```python
from build123d import *

# Parameters (mm, degrees)
SKETCH1_R           = 10
BOSS_EXTRUDE1_DEPTH = 2
SKETCH2_R           = 2.5
CUT_EXTRUDE1_DEPTH  = 2
SKETCH3_R           = 1
CUT_EXTRUDE2_DEPTH  = 2


with BuildPart() as part:
    # Sketch1 → Boss-Extrude1 (new body)
    with BuildSketch(Plane(origin=(0, 0, 0), x_dir=(1, 0, 0), z_dir=(0, 1, 0))):
        with Locations(Location((0, 0, 0), (0, 0, 270))):
            Circle(SKETCH1_R)
    extrude(amount=BOSS_EXTRUDE1_DEPTH)

    # Sketch2 → Cut-Extrude1 (cut)
    with BuildSketch(Plane(origin=(0, 2, 0), x_dir=(1, 0, 0), z_dir=(0, 1, 0))):
        with Locations(Location((0, 0, 0), (0, 0, 270))):
            Circle(SKETCH2_R)
    extrude(amount=-CUT_EXTRUDE1_DEPTH, mode=Mode.SUBTRACT)

    # Sketch3 → Cut-Extrude2 (cut)
    with BuildSketch(Plane(origin=(0, 2, 0), x_dir=(1, 0, 0), z_dir=(0, 1, 0))):
        with Locations(Location((7, 0, 0), (0, 0, 270))):
            Circle(SKETCH3_R)
        with Locations(Location((0, -7, 0), (0, 0, 270))):
            Circle(SKETCH3_R)
        with Locations(Location((-7, 0, 0), (0, 0, 270))):
            Circle(SKETCH3_R)
        with Locations(Location((0, 7, 0), (0, 0, 270))):
            Circle(SKETCH3_R)
    extrude(amount=-CUT_EXTRUDE2_DEPTH, mode=Mode.SUBTRACT)


solid = part.part
```
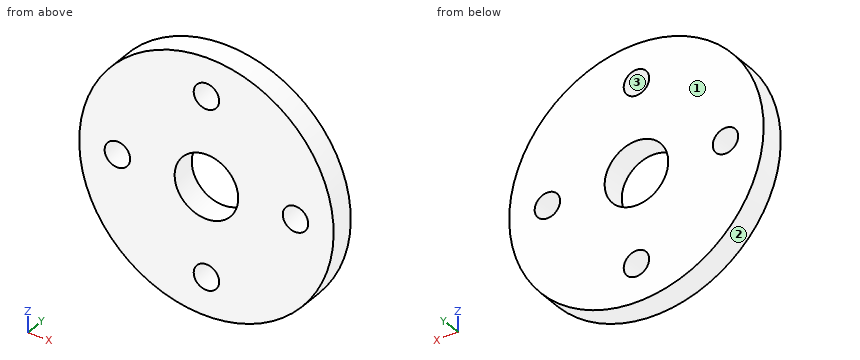
CAD build for the part. Positions are in the model's coordinates, mm. Face numbers are marked on the shaded views. Coordinates: 2 decimals unless noted, no trailing zeros. Write each loop counter-clockwise with the first axis right and the second up, starting at its lowest first coordinate (ties: lowest second). Pieces come first, ordered by that corner, then holes.
(1) Cut at A-A, the plane z = 0. List the corners of the cut face in (x, y), and give its area (3 significant figures).
(2) Cut at C-C, the plane y = 1.4. List the corners of the cut face in (x, z), and give its area (3 significant figures).
(3) Cut at D-D, the plane z = -7. List the corners of the cut face in (x, y), and give its area (3 significant figures).
(4) Two-plate mould, pull along X, no slides. Class the marked faces 1, 2 and 3: +X half, -X half, draft (parallel to the pull), parting line (faces both ways), or undercut.
(5) Drill centre lines: probe 1 along X at (y, z) = (0.9, 0); probe 2 along X at (y, z) = (1.2, 7); probe 3 along Z at (x, y) = (-2, 1.95). Where is each one in solid material? Low to high.
(6) Cut at B-B, the plane x = 0. List the corners of the cut face in (y, z), and give its area (3 significant figures).
(7) Flat gauge pin, fed straight in: pin 1 (1.2 mm diameter, centred on x = 0, z = -7, fed in from -Y). Where does the tip first touch, or does it go through?
Geometry says:
1. outline: (-10, 0) - (-8, 0) - (-8, 2) - (-10, 2) - close; (-6, 0) - (-2.5, 0) - (-2.5, 2) - (-6, 2) - close; (2.5, 0) - (6, 0) - (6, 2) - (2.5, 2) - close; (8, 0) - (10, 0) - (10, 2) - (8, 2) - close
1. area: 22.0 mm2
2. outline: circle Ø20 at (0, 0); hole circle Ø2 at (-7, 0); hole circle Ø5 at (0, 0); hole circle Ø2 at (0, -7); hole circle Ø2 at (0, 7); hole circle Ø2 at (7, 0)
2. area: 282 mm2
3. outline: (-7.14, 0) - (-1, 0) - (-1, 2) - (-7.14, 2) - close; (1, 0) - (7.14, 0) - (7.14, 2) - (1, 2) - close
3. area: 24.6 mm2
4. face 1: draft
4. face 2: parting line
4. face 3: undercut
5. probe 1: x = -10 to -8, -6 to -2.5, 2.5 to 6, 8 to 10
5. probe 2: x = -7.14 to -1, 1 to 7.14
5. probe 3: z = -9.8 to -1.5, 1.5 to 9.8
6. outline: (0, -10) - (2, -10) - (2, -8) - (0, -8) - close; (0, -6) - (2, -6) - (2, -2.5) - (0, -2.5) - close; (0, 2.5) - (2, 2.5) - (2, 6) - (0, 6) - close; (0, 8) - (2, 8) - (2, 10) - (0, 10) - close
6. area: 22.0 mm2
7. pin 1: passes through
